```python
from build123d import *

# Parameters (mm, degrees)
CROQUIS1_W              = 112
CROQUIS1_H              = 76
CROQUIS1_W_2            = 104
CROQUIS1_H_2            = 68
SALIENTE_EXTRUIR3_DEPTH = 1
CROQUIS2_W              = 112
CROQUIS2_H              = 1
SALIENTE_EXTRUIR4_DEPTH = 3
CROQUIS3_W              = 110
CROQUIS3_H              = 1
SALIENTE_EXTRUIR7_DEPTH = 1
CROQUIS5_W              = 110
CROQUIS5_H              = 1
SALIENTE_EXTRUIR8_DEPTH = 1


with BuildPart() as part:
    # Croquis1 → Saliente-Extruir3 (new body)
    with BuildSketch(Plane(origin=(0, 0, 0), x_dir=(1, 0, 0), z_dir=(0, 1, 0))):
        with Locations((56, 38)):
            Rectangle(CROQUIS1_W, CROQUIS1_H)
        with Locations((56, 38)):
            Rectangle(CROQUIS1_W_2, CROQUIS1_H_2, mode=Mode.SUBTRACT)
    extrude(amount=SALIENTE_EXTRUIR3_DEPTH)

    # Croquis2 → Saliente-Extruir4 (add)
    with BuildSketch(Plane(origin=(0, 1, 0), x_dir=(1, 0, 0), z_dir=(0, 1, 0))):
        with Locations((56, 75.5)):
            Rectangle(CROQUIS2_W, CROQUIS2_H)
        with Locations((56, 0.5)):
            Rectangle(CROQUIS2_W, CROQUIS2_H)
    extrude(amount=SALIENTE_EXTRUIR4_DEPTH)

    # Croquis3 → Saliente-Extruir7 (add)
    with BuildSketch(Plane(origin=(0, 0, -1), x_dir=(-1, 0, 0), z_dir=(0, 0, -1))):
        with Locations((-55, 3.5)):
            Rectangle(CROQUIS3_W, CROQUIS3_H)
    extrude(amount=SALIENTE_EXTRUIR7_DEPTH)

    # Croquis5 → Saliente-Extruir8 (add)
    with BuildSketch(Plane.XY.offset(-75)):
        with Locations((55, 3.5)):
            Rectangle(CROQUIS5_W, CROQUIS5_H)
    extrude(amount=SALIENTE_EXTRUIR8_DEPTH)


solid = part.part
```
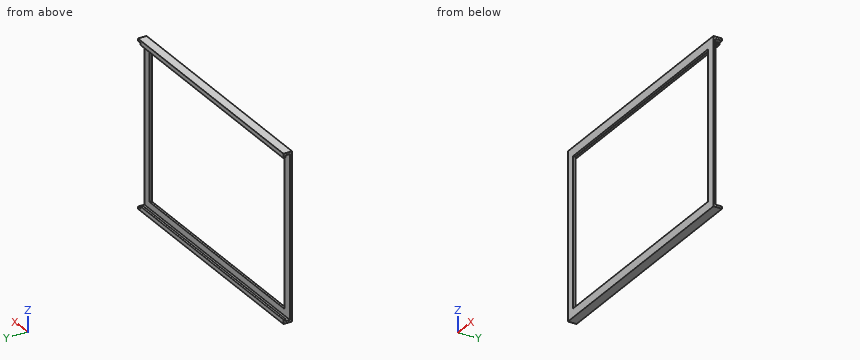
Build history of the part. All positions in model axes, mm. Round coordinates to 2 decimals unless told otherwise and drop trailing zeros. Order: outer loops, then holes, each group sorted by start corner. A loop starts at its lowest first (then second) coordinate and runs counter-clockwise, first axis right, second up. Notation, with made-up numbers: (30.25, 78) - (78.25, 78) arc R29 ccw to (78.25, 109) - close; hole circle Ø5 at (58.5, 62.5). An arc over 180 degrees is marked (long way). Use a Markdown table: item, result.
1) Saw through at B-B on y = 2. Write the cut outline in (x, z).
Recorded:
| item | result |
|---|---|
| outline | (0, -76) - (112, -76) - (112, -75) - (0, -75) - close; (0, -1) - (112, -1) - (112, 0) - (0, 0) - close |
2) Saw through at A-A on x = 59. Write the cut outline in (y, z).
Recorded:
| item | result |
|---|---|
| outline | (0, -76) - (4, -76) - (4, -74) - (3, -74) - (3, -75) - (1, -75) - (1, -72) - (0, -72) - close; (0, -4) - (1, -4) - (1, -1) - (3, -1) - (3, -2) - (4, -2) - (4, 0) - (0, 0) - close |
3) Saw through at C-C on z = -14.5. Write the cut outline in (x, y), and give its area (3 significant figures).
Recorded:
| item | result |
|---|---|
| outline | (0, 0) - (4, 0) - (4, 1) - (0, 1) - close; (108, 0) - (112, 0) - (112, 1) - (108, 1) - close |
| area | 8.00 mm² |
4) Wall check: L1, parallel to Z at x = 42, y = 1.4; L2, parallel to Z at x = 66, y = 3.4. Give the ranges that are in metal, low to high.
Recorded:
| item | result |
|---|---|
| L1 | z = -76 to -75, -1 to 0 |
| L2 | z = -76 to -74, -2 to 0 |
5) Flat gauge pins, fed straight in: pin 1 Ø1.5 at (y, z) = (2.5, -26) entering from +X; pin 2 Ø0.8 at (y, z) = (3.5, -1.5) entering from +X. Where does each tip first touch, or does it go through?
Recorded:
| item | result |
|---|---|
| pin 1 | passes through |
| pin 2 | stops at x = 110 |
